Check sheet for the modelled part. Datum: model origin and axes. Units: mm. Face numbers are marked on the shaded views. A direction names the side the tool comes from. Coordinates: 2 decimals unless noted, no trailing zeros. Write each loop counter-clockwise with the first axis right and the second up, starting at its lowest first coordinate (ties: lowest second). Pieces come first, ordered by that corner, then holes. Notation, with made-up numbers: (39.25, 72) - (71.25, 72) arc R7 ccw to (71.25, 83) - close; hole circle Ø2 at (37.25, 51). An arc over 180 degrees is marked (long way). Use one line per item in the form item = value. Start each with the question number.
1. Scan lines: line 1 along Y through (x, z) = (0, 18); line 2 along X through (y, z) = (-4, 7.5); line 3 along Z through (x, y) = (-16.5, 52). Record each from-to range of solid material in increasing order.
2. Go/stop test with flat-tipped pins: pin 1 Ø1.8 at (y, z) = (27.5, 53.5) entering from -X; pin 2 Ø6 at (x, z) = (6, 66) entering from -Y; pin 3 Ø1.1 at (y, z) = (27.5, 23) entering from +X; pin 4 Ø14.5 at (x, y) = (0, -75) entering from -Z. Record where each tip stops, or that it passes through.
3. Cross-section at D-D on z = 22. Record the boundary of the cut face in (x, y).
4. Tool access check on the marked faces 4, 5 and 6. Record the directions out of +Z, -Z, +X, -X, +Y, -Y that give a thin tool (end or side, any length) a straight path to the whole face; none if there is none.
5. Draft check along Y on the marked faces 1, 2 and 3. Enter one of: +Y half, -Y half, draft (parallel to the pull), parting line (faces both ways), or undercut.
6. Cross-section at C-C on y = -23.5. Record the boundary of the cut face in (x, z), then the cut area to 3 significant figures.
7. Cross-section at A-A on z = 43. Record the boundary of the cut face in (x, y), then the cut area to 3 significant figures.
8. Cross-section at B-B on x = 75. Record the boundary of the cut face in (y, z), then the cut area to 3 significant figures.
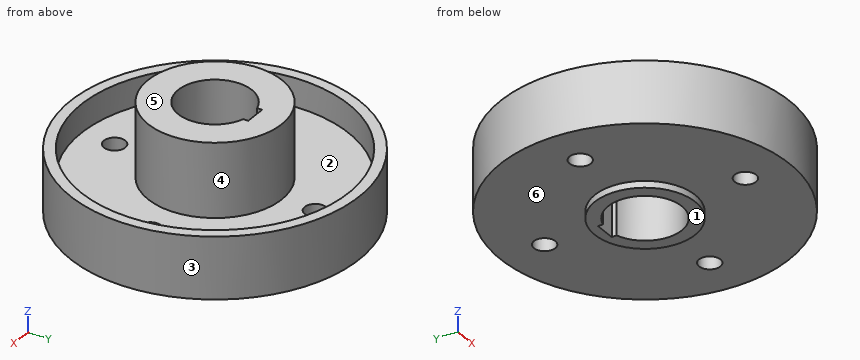
```python
from build123d import *

# Parameters (mm, degrees)
SKETCH1_R           = 108
BOSS_EXTRUDE1_DEPTH = 25
SKETCH2_R           = 108
SKETCH2_R_2         = 100
BOSS_EXTRUDE2_DEPTH = 21
SKETCH3_R           = 50
SKETCH3_R_2         = 27.5
BOSS_EXTRUDE3_DEPTH = 55
SKETCH4_R           = 37.5
BOSS_EXTRUDE4_DEPTH = 5
SKETCH6_R           = 27.5
CUT_EXTRUDE1_DEPTH  = 31
SKETCH7_R           = 8
CUT_EXTRUDE2_DEPTH  = 31
SKETCH9_W           = 16
SKETCH9_H           = 30
CUT_EXTRUDE4_DEPTH  = 86


with BuildPart() as part:
    # Sketch1 → Boss-Extrude1 (new body)
    with BuildSketch(Plane.XY):
        Circle(SKETCH1_R)
    extrude(amount=BOSS_EXTRUDE1_DEPTH)

    # Sketch2 → Boss-Extrude2 (add)
    with BuildSketch(Plane.XY.offset(25)):
        Circle(SKETCH2_R)
        Circle(SKETCH2_R_2, mode=Mode.SUBTRACT)
    extrude(amount=BOSS_EXTRUDE2_DEPTH)

    # Sketch3 → Boss-Extrude3 (add)
    with BuildSketch(Plane.XY.offset(25)):
        Circle(SKETCH3_R)
        Circle(SKETCH3_R_2, mode=Mode.SUBTRACT)
    extrude(amount=BOSS_EXTRUDE3_DEPTH)

    # Sketch4 → Boss-Extrude4 (add)
    with BuildSketch(Plane(origin=(0, 0, 0), x_dir=(-1, 0, 0), z_dir=(0, 0, -1))):
        Circle(SKETCH4_R)
    extrude(amount=BOSS_EXTRUDE4_DEPTH)

    # Sketch6 → Cut-Extrude1 (cut, through all)
    with BuildSketch(Plane.XY.offset(25)):
        Circle(SKETCH6_R)
    extrude(amount=-CUT_EXTRUDE1_DEPTH, mode=Mode.SUBTRACT)

    # Sketch7 → Cut-Extrude2 (cut, through all)
    with BuildSketch(Plane.XY.offset(25)):
        with Locations((0, 75)):
            Circle(SKETCH7_R)
        with Locations((75, 0)):
            Circle(SKETCH7_R)
        with Locations((0, -75)):
            Circle(SKETCH7_R)
        with Locations((-75, 0)):
            Circle(SKETCH7_R)
    extrude(amount=-CUT_EXTRUDE2_DEPTH, mode=Mode.SUBTRACT)

    # Sketch9 → Cut-Extrude4 (cut, through all)
    with BuildSketch(Plane.XY.offset(80)):
        with Locations((0, 15)):
            Rectangle(SKETCH9_W, SKETCH9_H)
    extrude(amount=-CUT_EXTRUDE4_DEPTH, mode=Mode.SUBTRACT)


solid = part.part
```
Final values:
q1.line_1 = -108 to -83, -67 to -27.5, 30 to 67, 83 to 108
q1.line_2 = -107.93 to -81.93, -68.07 to -27.21, 27.21 to 68.07, 81.93 to 107.93
q1.line_3 = 0 to 25
q2.pin_1 = -42.34
q2.pin_2 = -49.91
q2.pin_3 = 104.58
q2.pin_4 = through
q3.outline = circle Ø216 at (0, 0); hole circle Ø16 at (-75, 0); hole circle Ø16 at (0, -75); hole (-8, 26.31) arc R27.5 ccw (long way) to (8, 26.31) - (8, 30) - (-8, 30) - close; hole circle Ø16 at (0, 75); hole circle Ø16 at (75, 0)
q4.face_4 = +Z
q4.face_5 = +Z, +X, -X, +Y, -Y
q4.face_6 = -Z
q5.face_1 = draft
q5.face_2 = undercut
q5.face_3 = parting line
q6.outline = (-105.41, 0) - (-29.22, 0) - (-29.22, -5) - (-14.28, -5) - (-14.28, 80) - (-44.13, 80) - (-44.13, 25) - (-97.2, 25) - (-97.2, 46) - (-105.41, 46) - close; (14.28, -5) - (29.22, -5) - (29.22, 0) - (105.41, 0) - (105.41, 46) - (97.2, 46) - (97.2, 25) - (44.13, 25) - (44.13, 80) - (14.28, 80) - close
q6.area = 8,330 mm²
q7.outline = circle Ø216 at (0, 0); circle Ø100 at (0, 0); hole circle Ø200 at (0, 0); hole (-8, 26.31) arc R27.5 ccw (long way) to (8, 26.31) - (8, 30) - (-8, 30) - close
q7.area = 10,700 mm²
q8.outline = (-77.71, 0) - (-8, 0) - (-8, 25) - (-66.14, 25) - (-66.14, 46) - (-77.71, 46) - close; (8, 0) - (77.71, 0) - (77.71, 46) - (66.14, 46) - (66.14, 25) - (8, 25) - close
q8.area = 3,970 mm²
